Verification items for this drawing (mm, ordinates from the low corner). Coordinates: 2 decimals unless noted, no trailing zeros. Loops run counter-clockwise (first coordinate to the right, second up) from the corner with the lowest first, then second, coordinate; pieces in that order, holes last. Notation, with made-up numbers: M 71,-19.5 L 92,-19.5 A12 cw 92,-1.5 Z; hole C -1.75,69.5 d4. An arc over 180 degrees is marked long. Return JSON: item names as keys, results as strings.
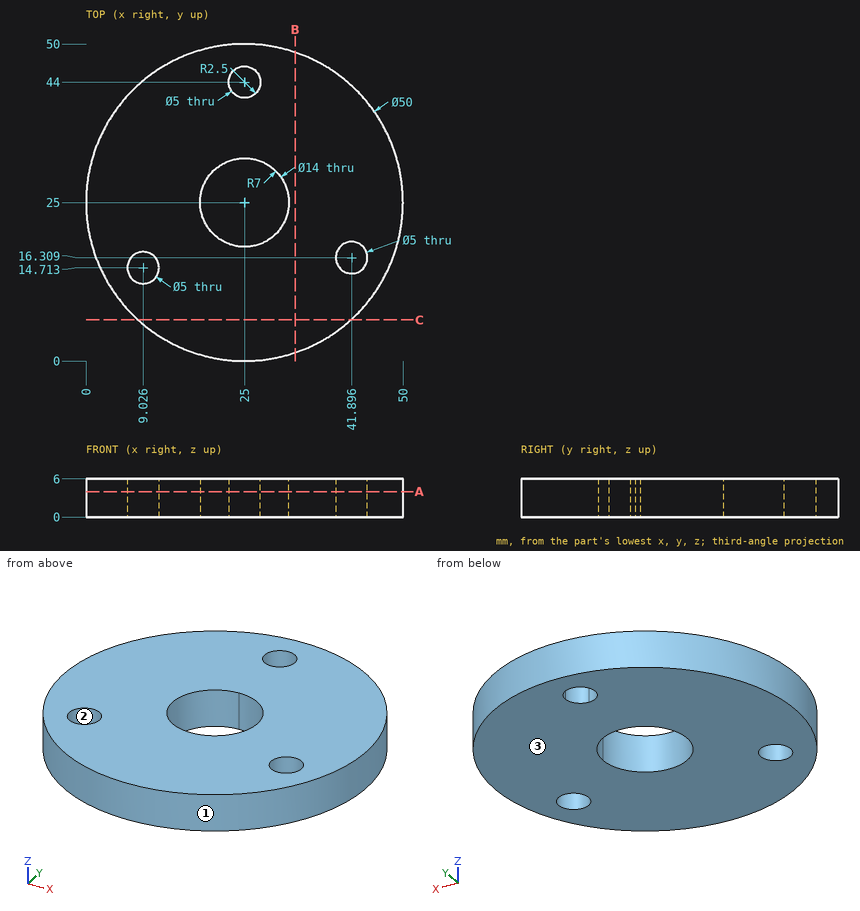
1) Section check C-C on y = 6.5. Record the cut outline in (x, z) (1 decimal), then the cut area to 3 significant figures.
Answers:
{"outline": "M 8.2,0 L 41.8,0 L 41.8,6 L 8.2,6 Z", "area": "202 mm²"}
2) Section check A-A on z = 4. Record the cut outline in (x, y) (1 decimal), then the cut area to 3 significant figures.
Answers:
{"outline": "C 25,25 d50; hole C 9,14.7 d5; hole C 25,44 d5; hole M 25,32 A7 ccw long 32,25 A7 ccw Z; hole C 41.9,16.3 d5", "area": "1,750 mm²"}
3) Go/stop test with flat-tipped pins: pin 1 Ø1 at (y, z) = (26.5, 3.5) entering from -X; pin 2 Ø3 at (y, z) = (41.5, 4.5) entering from +X; pin 3 Ø1 at (y, z) = (8.5, 2.5) entering from +X. Record where each tip stops, or that it passes through.
Answers:
{"pin 1": "x = 0.02", "pin 2": "x = 45", "pin 3": "x = 44.21"}
4) Scan lines: line 1 along Y through (x, z) = (25, 1.3); line 2 along X through (y, z) = (27, 3.45); line 3 along X through (y, z) = (27.5, 2) (1 decimal). Record each from-to range of solid material in increasing order. Write a range as [from, to].
Answers:
{"line 1": "[0, 18], [32, 41.5], [46.5, 50]", "line 2": "[0.08, 18.29], [31.71, 49.92]", "line 3": "[0.1, 18.5], [31.5, 49.9]"}
5) Draft check along Y on the marked faces 1, 2 and 3. Enter one of: +Y half, -Y half, draft (parallel to the pull), parting line (faces both ways), or undercut.
Answers:
{"face 1": "parting line", "face 2": "undercut", "face 3": "draft"}
6) Section check B-B on x = 33. Record the cut outline in (y, z) (1 decimal), then the cut area to 3 significant figures.
Answers:
{"outline": "M 1.3,0 L 48.7,0 L 48.7,6 L 1.3,6 Z", "area": "284 mm²"}
